Can you work these out from the model? Positions are in its coordinate system, mm. A direction names the side the tool comes from. Give positions to 0.01 mm unless a question says otherwise; leave off trailing zeros. Order: outer loops, then holes, each group sorted by start corner. A loop starts at its lowest first (then second) coordinate and runs counter-clockwise, first axis right, second up. Notation, with made-up numbers: M -4.5,88 L 3.5,88 A37 cw 3.5,125 Z; hole C 17,75.5 d11. An arc over 180 degrees is marked long. Use one line per item in the form item = value. Start each with the question number.
1. Will this pin go through, and if not, where does the flat tip stop? P1, Ø1, axis at y = -2, z = 2, coming from the +X side.
2. We'd pull the mould along Y, two halves only. Please class faces 1 (the face through (18.06, -26.07, 1.57)), 2 (the face through (48.106, 28.791, 1.565)), 3 (the face through (-12.537, 3.505, 1.565)), 4 (the face through (44.324, 68.851, 1.565)): +Y half, -Y half, draft (parallel to the pull), parting line (faces both ways), or undercut.
3. I want a section at A-A, the plane x = 0. List the corners of the cut face in (y, z) for me (1 decimal), and give its area (3 significant figures).
4. I need wall thicknesses on L1, parallel to X at y = 4.5, z = 1.55; L2, parallel to Y at x = 45.72, z = 0.7; L3, parallel to Y at x = 45, z = 1.7. Which ranges of each line are inside material? Lowest first, please.
5. I want a section at D-D, the plane x = 45.72. Count the separate pieces of the cut face and the enclosed holes in it, and give its area (3 significant figures).
6. I want a section at C-C, the plane y = 0. List the corners of the cut face in (x, z) for me (1 decimal).
7. For faces 5 (the face through (36.281, -16.002, 1.565)), 6 (the face through (42.704, 36.598, 1.565)), which set-ups out of +Z, -Z, +X, -X, +Y, -Y let a thin tool reach every point of the face, with its end or its side?
8. I want a section at B-B, the plane y = 34. List the corners of the cut face in (x, z) for me (3 decimals).
```python
from build123d import *

# Parameters (mm, degrees)
SKETCH2_R           = 7.9375
SKETCH2_R_2         = 3.2639
SKETCH2_R_3         = 4.191
BOSS_EXTRUDE1_DEPTH = 3.175
FILLET3_R           = 1.905
FILLET4_R           = 6.35
BOSS_EXTRUDE2_START = -3.175
BOSS_EXTRUDE2_DEPTH = 3.175
CUT_EXTRUDE1_DEPTH  = 12.065
FILLET5_R           = 3.175


with BuildPart() as part:
    # Sketch2 → Boss-Extrude1 (new body)
    with BuildSketch(Plane.XY):
        with BuildLine():
            Line((22.709173353, -24.74146542), (50.237344688, -7.01528789))
            ThreePointArc((50.237344688, -7.01528789), (52.649254226, -4.648236557), (53.924522204, -1.51871084))
            ThreePointArc((53.924522204, -1.51871084), (57.106411985, 32.846575037), (54.035830718, 67.22198524))
            ThreePointArc((54.035830718, 67.22198524), (46.044632155, 72.608660166), (40.859194914, 64.485436554))
            Line((40.859194914, 64.485436554), (40.833827284, 64.453346951))
            ThreePointArc((40.833827284, 64.453346951), (30.975387354, 29.729811242), (-0.998479041, 12.979150429))
            ThreePointArc((-0.998479041, 12.979150429), (-12.595568055, 3.287395871), (-7.214067166, -10.835706769))
            Line((-7.214067166, -10.835706769), (13.567787564, -24.671601284))
            ThreePointArc((13.567787564, -24.671601284), (18.128061271, -26.069833859), (22.709173353, -24.74146542))
        make_face()
        Circle(SKETCH2_R, mode=Mode.SUBTRACT)
        with Locations((18.191828664, -17.726177531)):
            Circle(SKETCH2_R_2, mode=Mode.SUBTRACT)
        with Locations((45.72, 0)):
            Circle(SKETCH2_R_2, mode=Mode.SUBTRACT)
        with BuildLine():
            Line((40.584986991, 6.617553577), (21.318666843, -5.788581474))
            Line((21.318666843, -5.788581474), (11.074870198, -6.841239387))
            ThreePointArc((11.074870198, -6.841239387), (12.976194182, 1.036190528), (9.848859751, 8.512066016))
            ThreePointArc((9.848859751, 8.512066016), (23.445327069, 14.632175726), (34.749899024, 24.354640398))
            Line((34.749899024, 24.354640398), (40.584986991, 6.617553577))
        make_face(mode=Mode.SUBTRACT)
        with BuildLine():
            ThreePointArc((47.523781163, 56.501393309), (48.257752726, 32.370804269), (45.933946154, 8.34115665))
            Line((45.933946154, 8.34115665), (38.882442516, 29.775817606))
            ThreePointArc((38.882442516, 29.775817606), (45.039190515, 42.544935267), (47.523781163, 56.501393309))
        make_face(mode=Mode.SUBTRACT)
        with Locations((47.413333333, 66.018287029)):
            Circle(SKETCH2_R_3, mode=Mode.SUBTRACT)
    extrude(amount=BOSS_EXTRUDE1_DEPTH)

    # Fillet3
    fillet3_edges = [part.edges().sort_by_distance(p)[0] for p in [
        (45.933946154, 8.34115665, 1.5875),
        (47.523781163, 56.501393309, 1.5875),
    ]]
    fillet(fillet3_edges, radius=FILLET3_R)

    # Fillet4
    fillet4_edges = [part.edges().sort_by_distance(p)[0] for p in [
        (38.882442516, 29.775817606, 1.5875),
    ]]
    fillet(fillet4_edges, radius=FILLET4_R)

    # Sketch3 → Boss-Extrude2 (add)
    with BuildSketch(Plane.XY.offset(3.175).offset(BOSS_EXTRUDE2_START)):
        with BuildLine():
            ThreePointArc((37.967247274, 14.574773228), (38.850624387, 9.974362656), (38.539279751, 5.300264126))
            Line((38.539279751, 5.300264126), (40.584986991, 6.617553577))
            Line((40.584986991, 6.617553577), (37.967247274, 14.574773228))
        make_face()
        with BuildLine():
            ThreePointArc((14.005375904, -6.540099084), (13.004272705, -4.28056917), (12.890798124, -1.811802966))
            ThreePointArc((12.890798124, -1.811802966), (12.243860592, -4.42076736), (11.074870198, -6.841239387))
            Line((11.074870198, -6.841239387), (14.005375904, -6.540099084))
        make_face()
        with BuildLine():
            ThreePointArc((9.848859751, 8.512066016), (12.486736073, 3.679229335), (12.890798124, -1.811802966))
            ThreePointArc((12.890798124, -1.811802966), (16.379474961, 7.582660649), (23.480082515, 14.654307207))
            ThreePointArc((23.480082515, 14.654307207), (16.886076234, 11.091387544), (9.848859751, 8.512066016))
        make_face()
    extrude(amount=BOSS_EXTRUDE2_DEPTH)

    # Sketch4 → Cut-Extrude1 (cut)
    with BuildSketch(Plane.XY):
        with BuildLine():
            Line((38.539279751, 5.300264126), (24.727997063, 1.47053375))
            ThreePointArc((24.727997063, 1.47053375), (25.836206507, -0.508508416), (26.220294441, -2.743953008))
            ThreePointArc((26.220294441, -2.743953008), (24.044282761, -7.68479904), (18.930249644, -9.41501626))
            ThreePointArc((18.930249644, -9.41501626), (30.477911362, -6.56779892), (37.848176473, 2.766778194))
            ThreePointArc((37.848176473, 2.766778194), (38.239149826, 4.021130685), (38.539279751, 5.300264126))
        make_face()
        with BuildLine():
            ThreePointArc((24.727997063, 1.47053375), (17.733373474, 3.709866579), (12.890798123, -1.811802972))
            Line((12.890798123, -1.811802972), (24.727997063, 1.47053375))
        make_face()
        with BuildLine():
            Line((24.727997063, 1.47053375), (12.890798123, -1.811802972))
            ThreePointArc((12.890798123, -1.811802972), (14.27873169, -6.909589201), (18.930249644, -9.41501626))
            ThreePointArc((18.930249644, -9.41501626), (24.044282761, -7.68479904), (26.220294441, -2.743953008))
            ThreePointArc((26.220294441, -2.743953008), (25.836206507, -0.508508416), (24.727997063, 1.47053375))
        make_face()
    extrude(amount=CUT_EXTRUDE1_DEPTH, mode=Mode.SUBTRACT)

    # Fillet5
    fillet5_edges = [part.edges().sort_by_distance(p)[0] for p in [
        (34.749899024, 24.354640398, 1.5875),
    ]]
    fillet(fillet5_edges, radius=FILLET5_R)


solid = part.part
```
Check result:
q1.P1 = 53.93
q2.face_1 = -Y half
q2.face_2 = undercut
q2.face_3 = parting line
q2.face_4 = undercut
q3.outline = M -15.6,0 L -7.9,0 L -7.9,3.2 L -15.6,3.2 Z; M 7.9,0 L 13.1,0 L 13.1,3.2 L 7.9,3.2 Z
q3.area = 40.7 mm2
q4.L1 = -12.21 to -6.54, 6.54 to 14.71, 38.36 to 54.94
q4.L2 = -9.92 to -3.26, 3.26 to 14.91, 42.51 to 62.18, 69.85 to 72.53
q4.L3 = -10.39 to -3.18, 3.18 to 14.84, 41.99 to 62.59, 69.44 to 72.3
q5.separate_pieces = 4
q5.enclosed_holes = 0
q5.area = 129 mm2
q6.outline = M -13,0 L -7.9,0 L -7.9,3.2 L -13,3.2 Z; M 7.9,0 L 13.2,0 L 13.2,3.2 L 7.9,3.2 Z; M 36.6,0 L 42.5,0 L 42.5,3.2 L 36.6,3.2 Z; M 49,0 L 54.2,0 L 54.2,3.2 L 49,3.2 Z
q7.face_5 = +Z, -Z, +X, -Y
q7.face_6 = +Z, -Z
q8.outline = M 34.055,0 L 41.406,0 L 41.406,3.175 L 34.055,3.175 Z; M 48.305,0 L 57.105,0 L 57.105,3.175 L 48.305,3.175 Z
